Geometry: final body of the model. Coordinates: model frame, mm. A direction names the side the tool comes from. Coordinates: 2 decimals unless noted, no trailing zeros. Loops run counter-clockwise (first coordinate to the right, second up) from the corner with the lowest first, then second, coordinate; pieces in that order, holes last. Notation, with made-up numbers: (22.5, 32.5) - (72.5, 32.5) arc R14 cw to (72.5, 45.5) - close; hole circle Ø6 at (36, -17.75). An arc over 180 degrees is marked (long way). Put each result on its own line as item: value. Start each with the question number.
1) Draft query along Y for faces 3 (the cylindrical face through (60.015, -4.053, 3.479)), 4 (the flat face through (6, 10, 2)), 5 (the flat face through (6.5, -7.61, 4.24)), 6 (the cylindrical face through (0.57, -9.4, 2.54)). Return one class per face: +Y half, -Y half, draft (parallel to the pull), parting line (faces both ways), or undercut.
2) Section B-B on x = 5. Output: boundary loops of the cut face in (y, z).
3) Section D-D on z = 4.2. Count the separate pieces of the cut face and the enclosed holes in it, and give its area (3 significant figures).
4) Section A-A on y = 0. Output: boundary loops of the cut face in (x, z), and give its area (3 significant figures).
5) Section C-C on x = 32.5. Output: boundary loops of the cut face in (y, z).
6) Reachability of faces 1 (the cylindrical face through (3.45, -5.07, 1.73)), 2 (the flat face through (61.77, -3.03, 3.48)) from +Z, -Z, +X, -X, +Y, -Y: full face, straight path, thin tool, end or side. Return the list, or none.
7) Contact query for flat-ended pins moving along their axis: pin 1 Ø3 at (y, z) = (0.5, 3) entering from +X; pin 2 Ø4 at (x, y) = (24, 3.5) entering from +Z; pin 3 Ø1.2 at (y, z) = (-2, 2.5) entering from +X; pin 4 Ø5 at (x, y) = (5, -5) entering from +Z. Output: stop coordinate, or through.
8) Material intervals for line 1 along Y through (x, z) = (5, 2.55); line 2 along Z through (x, y) = (23, 3); line 3 along X through (y, z) = (-1.25, 2.65), sorted ascending. Write a range as from..to.
Autodesk Inventor part; units mm, degrees
ref_plane "YZ Plane" through (0, 0, 0) normal (1, 0, 0) x (0, 1, 0)
ref_plane "XZ Plane" through (0, 0, 0) normal (0, 1, 0) x (-1, 0, 0)
ref_plane "XY Plane" through (0, 0, 0) normal (0, 0, 1) x (1, 0, 0)
sketch "スケッチ1" plane through (0, 0, 0) normal (0, 0, 1) x (1, 0, 0)
  circle A0 centre (5, 5) radius 1.55
  circle A1 centre (5, -5) radius 1.55
  line L0 (0, 0) -> (60, 0) construction
  circle A2 centre (60, 0) radius 1.55
  line L1 (0, 10) -> (0, -10)
  line L2 (0, -10) -> (10, -10)
  line L3 (10, -10) -> (60.4762, -5.9811)
  line L4 (10, 10) -> (60.4762, 5.9811)
  arc A3 (60.4762, -5.9811) -> (60.4762, 5.9811) centre (60, 0) ccw
  line L5 (55.0583, -3.4029) -> (11, -6.9109)
  line L6 (55.0583, 3.4029) -> (11, 6.9109)
  arc A4 (55.0583, 3.4029) -> (55.0583, -3.4029) centre (60, 0) ccw
  line L7 (11, -6.9109) -> (11, 6.9109)
  line L8 (5, -5) -> (5, 5)
  line L9 (0, 10) -> (10, 10)
  line L10 (8.01, 6.7378) -> (8.01, 3.2622)
  line L11 (8.01, 3.2622) -> (5, 1.5244)
  line L12 (5, 1.5244) -> (1.99, 3.2622)
  line L13 (1.99, 3.2622) -> (1.99, 6.7378)
  line L14 (1.99, 6.7378) -> (5, 8.4756)
  line L15 (5, 8.4756) -> (8.01, 6.7378)
  arc A5 (4.0907, 2.0494) -> (5.9093, 2.0494) centre (5, 2.5744) ccw
  arc A6 (7.1007, 2.7372) -> (8.01, 4.3122) centre (7.1007, 3.7872) ccw
  arc A7 (8.01, 5.6878) -> (7.1007, 7.2628) centre (7.1007, 6.2128) ccw
  arc A8 (5.9093, 7.9506) -> (4.0907, 7.9506) centre (5, 7.4256) ccw
  arc A9 (2.8993, 7.2628) -> (1.99, 5.6878) centre (2.8993, 6.2128) ccw
  arc A10 (1.99, 4.3122) -> (2.8993, 2.7372) centre (2.8993, 3.7872) ccw
  line L16 (8.01, -6.7378) -> (8.01, -3.2622)
  line L17 (8.01, -3.2622) -> (5, -1.5244)
  line L18 (5, -1.5244) -> (1.99, -3.2622)
  line L19 (1.99, -3.2622) -> (1.99, -6.7378)
  line L20 (1.99, -6.7378) -> (5, -8.4756)
  line L21 (5, -8.4756) -> (8.01, -6.7378)
  arc A11 (5.9093, -2.0494) -> (4.0907, -2.0494) centre (5, -2.5744) ccw
  arc A12 (8.01, -4.3122) -> (7.1007, -2.7372) centre (7.1007, -3.7872) ccw
  arc A13 (7.1007, -7.2628) -> (8.01, -5.6878) centre (7.1007, -6.2128) ccw
  arc A14 (4.0907, -7.9506) -> (5.9093, -7.9506) centre (5, -7.4256) ccw
  arc A15 (1.99, -5.6878) -> (2.8993, -7.2628) centre (2.8993, -6.2128) ccw
  arc A16 (2.8993, -2.7372) -> (1.99, -4.3122) centre (2.8993, -3.7872) ccw
  circle A17 centre (60, 0) radius 1.55
  line L22 (63.51, 2.0265) -> (63.51, -2.0265)
  line L23 (63.51, -2.0265) -> (60, -4.053)
  line L24 (60, -4.053) -> (56.49, -2.0265)
  line L25 (56.49, -2.0265) -> (56.49, 2.0265)
  line L26 (56.49, 2.0265) -> (60, 4.053)
  line L27 (60, 4.053) -> (63.51, 2.0265)
  arc A18 (59.0907, -3.528) -> (60.9093, -3.528) centre (60, -3.003) ccw
  arc A19 (62.6007, -2.5515) -> (63.51, -0.9765) centre (62.6007, -1.5015) ccw
  arc A20 (63.51, 0.9765) -> (62.6007, 2.5515) centre (62.6007, 1.5015) ccw
  arc A21 (60.9093, 3.528) -> (59.0907, 3.528) centre (60, 3.003) ccw
  arc A22 (57.3993, 2.5515) -> (56.49, 0.9765) centre (57.3993, 1.5015) ccw
  arc A23 (56.49, -0.9765) -> (57.3993, -2.5515) centre (57.3993, -1.5015) ccw
  line L28 (60, 4.053) -> (60, -4.053) construction
  point P0 (5, 0)
  point P1 (8.01, 3.2622)
  point P2 (8.01, 6.7378)
  point P3 (5, 8.4756)
  point P4 (1.99, 6.7378)
  point P5 (2.8993, 2.7372)
  point P6 (1.99, 4.3122)
  point P7 (1.99, 5.6878)
  point P8 (2.8993, 7.2628)
  point P9 (4.0907, 7.9506)
  point P10 (5.9093, 7.9506)
  point P11 (7.1007, 7.2628)
  point P12 (8.01, 5.6878)
  point P13 (8.01, 4.3122)
  point P14 (7.1007, 2.7372)
  point P15 (7.1007, -2.7372)
  point P16 (8.01, -4.3122)
  point P17 (8.01, -5.6878)
  point P18 (7.1007, -7.2628)
  point P19 (5.9093, -7.9506)
  point P20 (4.0907, -7.9506)
  point P21 (2.8993, -7.2628)
  point P22 (1.99, -5.6878)
  point P23 (1.99, -4.3122)
  point P24 (2.8993, -2.7372)
  point P25 (1.99, -6.7378)
  point P26 (5, -8.4756)
  point P27 (56.49, 2.0265)
  point P28 (56.49, -2.0265)
  point P29 (62.6007, -2.5515)
  point P30 (57.3993, -2.5515)
  point P31 (56.49, -0.9765)
  point P32 (56.49, 0.9765)
  point P33 (57.3993, 2.5515)
  point P34 (59.0907, 3.528)
  point P35 (60.9093, 3.528)
  point P36 (62.6007, 2.5515)
  point P37 (63.51, 0.9765)
  point P38 (63.51, -0.9765)
  dimension "d0" = 10
  dimension "d1" = 3.1
  dimension "d2" = 3.1
  dimension "d3" = 60
  dimension "d4" = 6
  dimension "d33" = 3
  dimension "d34" = 6
  dimension "d35" = 6
  dimension "d40" = 20
  dimension "d41" = 5
  dimension "d42" = 10
  dimension "d43" = 6.02
  dimension "d44" = 2.1
  dimension "d47" = 360
  dimension "d57" = 3.1
  dimension "d58" = 7.02
  dimension "d59" = 2.1
  dimension "d60" = 360
extrude "押し出し1" add sketch "スケッチ1" along normal blind 5 contours L9 L4 A3 L3 L2 L1
extrude "押し出し5" add sketch "スケッチ1" along normal blind 3.5 contours L12 L13 L14 L15 L10 L11 | L11 A5 | A11 L17 | L17 L16 L21 L20 L19 L18 | L18 A11 | A5 L12 | L11 A6 | A10 L12 | A12 L17 | L18 A16 | L10 A6 | A10 L13 | A12 L16 | L19 A16 | L10 A7 | A9 L13 | A13 L16 | L19 A15 | L15 A7 | A9 L14 | A13 L21 | L20 A15 | L15 A8 | A8 L14 | A14 L21 | L20 A14
extrude "押し出し6" add sketch "スケッチ1" along normal blind 2 contours A20 L22 | L22 L23 L24 L25 L26 L27 | L27 A20 | A19 L22 | L27 A21 | A19 L23 | L26 A21 | A18 L23 | L26 A22 | A18 L24 | L25 A22 | A23 L24 | L25 A23
extrude "押し出し7" add sketch "スケッチ1" along normal blind 1 contours L5 L7 L6 A4
fillet "フィレット2" radius 2 6 edges at (11, 6.9109, 3) (11, -6.9109, 3) (55.0583, 3.4029, 3) (55.0583, -3.4029, 3) (0, -10, 2.5) (0, 10, 2.5)
properties part number "Trunk_vertical_frame_05" material "アセタール樹脂、黒"
Answer block:
1. face 3: undercut
1. face 4: +Y half
1. face 5: undercut
1. face 6: -Y half
2. outline: (-10, 0) - (-6.55, 0) - (-6.55, 3.5) - (-8.48, 3.5) - (-8.48, 5) - (-10, 5) - close; (-3.45, 0) - (3.45, 0) - (3.45, 3.5) - (1.52, 3.5) - (1.52, 5) - (-1.52, 5) - (-1.52, 3.5) - (-3.45, 3.5) - close; (6.55, 0) - (10, 0) - (10, 5) - (8.48, 5) - (8.48, 3.5) - (6.55, 3.5) - close
3. separate pieces: 1
3. enclosed holes: 4
3. area: 502 mm²
4. outline: (0, 0) - (58.45, 0) - (58.45, 2) - (56.49, 2) - (56.49, 5) - (54, 5) - (54, 1) - (11, 1) - (11, 5) - (0, 5) - close; (61.55, 0) - (66, 0) - (66, 5) - (63.51, 5) - (63.51, 2) - (61.55, 2) - close
4. area: 131 mm²
5. outline: (-8.21, 0) - (8.21, 0) - (8.21, 5) - (5.2, 5) - (5.2, 1) - (-5.2, 1) - (-5.2, 5) - (-8.21, 5) - close
6. face 1: +Z, -Z
6. face 2: +Z
7. pin 1: stops at x = 66
7. pin 2: stops at z = 1
7. pin 3: stops at x = 65.83
7. pin 4: stops at z = 3.5
8. line 1: y = -10..-6.55, -3.45..3.45, 6.55..10
8. line 2: z = 0..1
8. line 3: x = 0..11, 54.13..56.38, 63.62..65.87
